```python
from build123d import *

# Parameters (mm, degrees)
SKETCH1_W           = 47
SKETCH1_H           = 47
SKETCH1_W_2         = 6.040926981
SKETCH1_H_2         = 17.482076569
SKETCH1_W_3         = 3.189765803
SKETCH1_H_3         = 10.04776228
BOSS_EXTRUDE2_DEPTH = 2
SKETCH6_R           = 34.5
SKETCH6_W           = 3.189765803
SKETCH6_H           = 10.04776228
SKETCH6_W_2         = 6.040926981
SKETCH6_H_2         = 17.482076569
BOSS_EXTRUDE4_DEPTH = 1


with BuildPart() as part:
    # Sketch1 → Boss-Extrude2 (new body)
    with BuildSketch(Plane(origin=(0, 0, 0), x_dir=(1, 0, 0), z_dir=(0, 1, 0))):
        Rectangle(SKETCH1_W, SKETCH1_H)
        with Locations((-16.490815369, -14.078790897)):
            Rectangle(SKETCH1_W_2, SKETCH1_H_2, mode=Mode.SUBTRACT)
        with Locations((-13.840536858, 17.764090865)):
            Rectangle(SKETCH1_W_3, SKETCH1_H_3, mode=Mode.SUBTRACT)
    extrude(amount=BOSS_EXTRUDE2_DEPTH)

    # Sketch6 → Boss-Extrude4 (add)
    with BuildSketch(Plane(origin=(0, 2, 0), x_dir=(1, 0, 0), z_dir=(0, 1, 0))):
        with Locations(Location((0, 0, 0), (0, 0, 270))):
            Circle(SKETCH6_R)
        with Locations((-13.840536858, 17.764090865)):
            Rectangle(SKETCH6_W, SKETCH6_H, mode=Mode.SUBTRACT)
        with Locations((-16.490815369, -14.078790897)):
            Rectangle(SKETCH6_W_2, SKETCH6_H_2, mode=Mode.SUBTRACT)
    extrude(amount=BOSS_EXTRUDE4_DEPTH)


solid = part.part
```
Here's how the part is built. I have some questions about the finished solid (model axes, mm). A direction names the side the tool comes from. Coordinates: 2 decimals unless noted, no trailing zeros. Order: outer loops, then holes, each group sorted by start corner. A loop starts at its lowest first (then second) coordinate and runs counter-clockwise, first axis right, second up. Notation, with made-up numbers: (-5, 64) -> (16, 64) arc R29 cw to (16, 96) -> close; hole circle Ø5 at (41.5, 48.5). An arc over 180 degrees is marked (long way). Return JSON: item names as keys, results as strings.
1) If we section it at B-B on z = 8.5: List the corners of the cut face in (x, y) for me, plus the area to 3 significant figures.
Conclusion:
{"outline": "(-33.44, 2) -> (-23.5, 2) -> (-23.5, 0) -> (-19.51, 0) -> (-19.51, 3) -> (-33.44, 3) -> close; (-13.47, 0) -> (23.5, 0) -> (23.5, 2) -> (33.44, 2) -> (33.44, 3) -> (-13.47, 3) -> close", "area": "143 mm²"}
2) On a 3-axis mill with a long thin cutter (end or side, diameter ignored), from which of +Z, -Z, +X, -X, +Y, -Y can I reach the whole of each face in a straight line? I mean faces 4 (the flat face through (0, 1, -23.5)), 5 (the flat face through (23.5, 1, 0)), 6 (the flat face through (0, 0, 0)), 7 (the flat face through (-19.511, 1, 14)), 8 (the flat face through (0, 1, 23.5)). Say none if no direction works.
Conclusion:
{"face 4": "-Z, +X, -X, -Y", "face 5": "+Z, -Z, +X, -Y", "face 6": "+Z, -Z, +X, -X, -Y", "face 7": "+Y, -Y", "face 8": "+Z, +X, -X, -Y"}
3) If we section it at A-A on y = 2.55: List the corners of the cut face in (x, z) for me, plus the area to 3 significant figures.
Conclusion:
{"outline": "circle Ø69 at (0, 0); hole (-19.51, 5.34) -> (-13.47, 5.34) -> (-13.47, 22.82) -> (-19.51, 22.82) -> close; hole (-15.44, -22.79) -> (-12.25, -22.79) -> (-12.25, -12.74) -> (-15.44, -12.74) -> close", "area": "3,600 mm²"}
4) If I drill on probe 1 along X at (y, z) = (1.9, 6); probe 2 along X at (y, z) = (1.9, -19.5); probe 3 along Z at (x, y) = (-17, 1.55), over which ranges is the centre line in solid material (lowest first)?
Conclusion:
{"probe 1": "x = -23.5 to -19.51, -13.47 to 23.5", "probe 2": "x = -23.5 to -15.44, -12.25 to 23.5", "probe 3": "z = -23.5 to 5.34, 22.82 to 23.5"}
5) If we section it at D-D on x = 22: List the corners of the cut face in (y, z) for me.
Conclusion:
{"outline": "(0, -23.5) -> (2, -23.5) -> (2, -26.58) -> (3, -26.58) -> (3, 26.58) -> (2, 26.58) -> (2, 23.5) -> (0, 23.5) -> close"}
6) Thinking about a two-plate mould opening in X: for faces 1 (the flat face through (-23.5, 1, 0)), 2 (the flat face through (0, 3, 0)), 3 (the flat face through (-13.47, 1, 14)), which applies, +X half, -X half, draft (parallel to the pull), parting line (faces both ways), or undercut?
Conclusion:
{"face 1": "-X half", "face 2": "draft", "face 3": "undercut"}
7) If we section it at C-C on z = 0: List the corners of the cut face in (x, y) for me.
Conclusion:
{"outline": "(-34.5, 2) -> (-23.5, 2) -> (-23.5, 0) -> (23.5, 0) -> (23.5, 2) -> (34.5, 2) -> (34.5, 3) -> (-34.5, 3) -> close"}
8) I'm going to push flat-ended pins straight in: P1, Ø1, axis at x = -10, y = 1, coming from the +Z side; P2, Ø1.5, axis at x = -13, y = 1.5, coming from the -Z side; P3, Ø1.5, axis at x = 26.5, y = 1, coming from the -Z side; P4, Ø1.5, axis at y = 1, z = 14, coming from the -X side. Where does each tip first touch, or does it pass through?
Conclusion:
{"P1": "stops at z = 23.5", "P2": "stops at z = -32.18", "P3": "passes through", "P4": "stops at x = -23.5"}
